Design review of the part built by this model. Coordinates are the model's own, in mm. A direction names the side the tool comes from. Give positions to 0.01 mm unless a question says otherwise; leave off trailing zeros. Loops run counter-clockwise (first coordinate to the right, second up) from the corner with the lowest first, then second, coordinate; pieces in that order, holes last. Notation, with made-up numbers: M 77,75.25 L 96,75.25 A22 cw 96,89.25 Z; hole C 80,61.5 d5. An arc over 180 degrees is marked long. Answer as CSV lines item,"result".
```python
from build123d import *

# Parameters (mm, degrees)
SKETCH1_W           = 25.4
SKETCH1_H           = 25.4
BOSS_EXTRUDE1_DEPTH = 342.9
SHELL1_T            = -1.5875
SKETCH2_R           = 2.4892
CUT_EXTRUDE1_DEPTH  = 344.370048199


with BuildPart() as part:
    # Sketch1 → Boss-Extrude1 (new, symmetric)
    with BuildSketch(Plane.XY):
        Rectangle(SKETCH1_W, SKETCH1_H)
    extrude(amount=BOSS_EXTRUDE1_DEPTH, both=True)

    # Shell1
    shell1_openings = [part.faces().sort_by_distance(p)[0] for p in [
        (0, 0, 342.9),
        (0, 0, -342.9),
    ]]
    offset(amount=SHELL1_T, openings=shell1_openings, kind=Kind.INTERSECTION)

    # Sketch2 → Cut-Extrude1 (cut, symmetric)
    with BuildSketch(Plane(origin=(0, 0, 0), x_dir=(1, 0, 0), z_dir=(0, 1, 0))):
        with Locations(Location((0, -330.2, 0), (0, 0, 270))):
            Circle(SKETCH2_R)
        with Locations(Location((0, -317.5, 0), (0, 0, 270))):
            Circle(SKETCH2_R)
        with Locations(Location((0, -304.8, 0), (0, 0, 270))):
            Circle(SKETCH2_R)
        with Locations(Location((0, -292.1, 0), (0, 0, 270))):
            Circle(SKETCH2_R)
    cut_extrude1 = extrude(amount=CUT_EXTRUDE1_DEPTH, both=True, mode=Mode.SUBTRACT)

    # Mirror1: Cut-Extrude1 across plane
    add(cut_extrude1.mirror(Plane.XY), mode=Mode.SUBTRACT)


solid = part.part
```
1. For P1, Ø10, axis at x = -1.5, y = -1.5, coming from the -Z side, flat-tipped, find the tip position at first contact; note if it passes through.
Answer block:
P1,"through"
2. For faces 1 (the flat face through (12.7, 0, 5)), 2 (the flat face through (-11.112, 0, 5)), list the 3-axis set-ups (+Z, -Z, +X, -X, +Y, -Y) from which the entire face can be reached by the end or side of a thin tool; tool diameter is ignored.
Answer block:
face 1,"+Z, -Z, +X, +Y, -Y"
face 2,"+Z, -Z"
3. We need section C-C, the plane z = 12. Write out the cut boundary in (x, y), plus the area to 3 significant figures.
Answer block:
outline,"M -12.7,-12.7 L 12.7,-12.7 L 12.7,12.7 L -12.7,12.7 Z; hole M -11.11,-11.11 L 11.11,-11.11 L 11.11,11.11 L -11.11,11.11 Z"
area,"151 mm²"
4. To check wall thickness, follow L1, parallel to Y at x = 6.5, z = -181; L2, parallel to X at y = -11.7, z = -304.8. State the ranges of each line that lie inside material, in increasing order. Write a range as [from, to].
Answer block:
L1,"[-12.7, -11.11], [11.11, 12.7]"
L2,"[-12.7, -2.49], [2.49, 12.7]"
5. We need section A-A, the plane x = 6.75. Write out the cut boundary in (y, z), plus the area to 3 significant figures.
Answer block:
outline,"M -12.7,-342.9 L -11.11,-342.9 L -11.11,342.9 L -12.7,342.9 Z; M 11.11,-342.9 L 12.7,-342.9 L 12.7,342.9 L 11.11,342.9 Z"
area,"2,180 mm²"
6. The part is to be moulded in two halves that separate along X. For faces 3 (the flat face through (0, 11.112, 5)), 4 (the flat face through (-11.3, 0.1, 342.9)), 5 (the flat face through (-12.7, 0, 5)), say which applies: pulls with the +X half, pulls with the -X half, needs draft (parallel to the pull), parting line crosses it, or undercut.
Answer block:
face 3,"undercut"
face 4,"needs draft"
face 5,"pulls with the -X half"
